from build123d import *

# Parameters (mm, degrees)
BOSS_EXTRUDE2_DEPTH = 50
CUT_EXTRUDE1_REACH  = 175.469
SKETCH2_W           = 5
SKETCH2_H           = 40
SKETCH3_W           = 40
SKETCH3_H           = 5
CUT_EXTRUDE4_DEPTH  = 25
CUT_EXTRUDE5_REACH  = 148.615
SKETCH5_W           = 40
SKETCH5_H           = 5
CUT_EXTRUDE6_REACH  = 175.469
SKETCH6_W           = 5
SKETCH6_H           = 40
FILLET1_R           = 10
FILLET2_R           = 3
FILLET3_R           = 8
CUT_EXTRUDE7_REACH  = 146.893
CUT_EXTRUDE8_DEPTH  = 145.893467036
SKETCH10_W          = 50
SKETCH10_H          = 14.886309014
CUT_EXTRUDE9_DEPTH  = 145.893467036
CUT_EXTRUDE10_REACH = 110.938
SKETCH11_R          = 6
CUT_EXTRUDE11_REACH = 144.895
SKETCH12_R          = 6


with BuildPart() as part:
    # Sketch1 → Boss-Extrude2 (new body)
    with BuildSketch(Plane.XY):
        Polygon((5, -20.716112532), (5, 136.021274565), (-55, 64.51605901), (-55, -20.716112532), (-45, -20.716112532), (-45, 60.876356667), (-5, 108.546500371), (-5, -20.716112532), align=None)
    extrude(amount=BOSS_EXTRUDE2_DEPTH)

    # Cut-Extrude1: up to this plane
    cut_extrude1_end = Plane(origin=(5, 136.021274565, 50), z_dir=(0.7660444431189773, -0.6427876096865403, 0))
    # Sketch2 → Cut-Extrude1 (cut, up to the surface)
    with BuildSketch(Plane.XZ.offset(20.716112532), mode=Mode.PRIVATE) as cut_extrude1_sk1:
        with Locations((-52.5, 25)):
            Rectangle(SKETCH2_W, SKETCH2_H)
    cut_extrude1_tool1 = split(extrude(cut_extrude1_sk1.sketch, amount=-CUT_EXTRUDE1_REACH, mode=Mode.PRIVATE), bisect_by=cut_extrude1_end, keep=Keep.BOTH, mode=Mode.PRIVATE)
    add(cut_extrude1_tool1.solids().sort_by_distance((-52.5, -20.716113, 25))[0], mode=Mode.SUBTRACT)

    # Sketch3 → Cut-Extrude4 (cut)
    with BuildSketch(Plane(origin=(14.043282439, 16.736132299, 0), x_dir=(0, 0, -1), z_dir=(0.6427876096865403, 0.7660444431189773, 0))):
        with Locations((-25, 81.102567729)):
            Rectangle(SKETCH3_W, SKETCH3_H)
    extrude(amount=-CUT_EXTRUDE4_DEPTH, mode=Mode.SUBTRACT)

    # Cut-Extrude5: up to this plane
    cut_extrude5_end = Plane(origin=(5, -20.716112532, 50), z_dir=(-1, 0, 0))
    # Sketch5 → Cut-Extrude5 (cut, up to the surface)
    with BuildSketch(Plane(origin=(14.043282439, 16.736132299, 0), x_dir=(0, 0, -1), z_dir=(0.6427876096865403, 0.7660444431189773, 0)), mode=Mode.PRIVATE) as cut_extrude5_sk1:
        with Locations((-25, 81.102567729)):
            Rectangle(SKETCH5_W, SKETCH5_H)
    cut_extrude5_tool1 = split(extrude(cut_extrude5_sk1.sketch, amount=CUT_EXTRUDE5_REACH, mode=Mode.PRIVATE), bisect_by=cut_extrude5_end, keep=Keep.BOTH, mode=Mode.PRIVATE)
    add(cut_extrude5_tool1.solids().sort_by_distance((-48.084889, 68.867858, 25))[0], mode=Mode.SUBTRACT)

    # Cut-Extrude6: up to this plane
    cut_extrude6_end = Plane(origin=(-62.239468027, 48.109777846, 45), z_dir=(0.7660444431189773, -0.6427876096865403, 0))
    # Sketch6 → Cut-Extrude6 (cut, up to the surface)
    with BuildSketch(Plane.XZ.offset(20.716112532), mode=Mode.PRIVATE) as cut_extrude6_sk1:
        with Locations((2.5, 25)):
            Rectangle(SKETCH6_W, SKETCH6_H)
    cut_extrude6_tool1 = split(extrude(cut_extrude6_sk1.sketch, amount=-CUT_EXTRUDE6_REACH, mode=Mode.PRIVATE), bisect_by=cut_extrude6_end, keep=Keep.BOTH, mode=Mode.PRIVATE)
    add(cut_extrude6_tool1.solids().sort_by_distance((2.5, -20.716113, 25))[0], mode=Mode.SUBTRACT)

    # Fillet1
    fillet1_edges = [part.edges().sort_by_distance(p)[0] for p in [
        (-45, 60.876356667, 25),
        (-55, 64.51605901, 47.5),
        (-55, 64.51605901, 2.5),
        (-50, 62.696207838, 25),
    ]]
    fillet(fillet1_edges, radius=FILLET1_R)

    # Fillet2
    fillet2_edges = [part.edges().sort_by_distance(p)[0] for p in [
        (-5, 108.546500371, 25),
        (0, 122.283887468, 25),
    ]]
    fillet(fillet2_edges, radius=FILLET2_R)

    # Fillet3
    fillet3_edges = [part.edges().sort_by_distance(p)[0] for p in [
        (5, 136.021274565, 47.5),
        (5, 136.021274565, 2.5),
    ]]
    fillet(fillet3_edges, radius=FILLET3_R)

    # Cut-Extrude7: up to this face of the body (flat: up to its plane)
    cut_extrude7_end = Plane(part.part.faces().sort_by_distance((5, 46.662671339, 2.5))[0])
    # Sketch8 → Cut-Extrude7 (cut, up to the picked face)
    with BuildSketch(Plane.ZY.offset(55), mode=Mode.PRIVATE) as cut_extrude7_sk1:
        Polygon((0, -20.716112532), (25, 19.170196482), (50, -20.716112532), align=None)
    cut_extrude7_tool1 = split(extrude(cut_extrude7_sk1.sketch, amount=-CUT_EXTRUDE7_REACH, mode=Mode.PRIVATE), bisect_by=cut_extrude7_end, keep=Keep.BOTH, mode=Mode.PRIVATE)
    add(cut_extrude7_tool1.solids().sort_by(Axis((-55, -7.420676, 25), (1, 0, 0)))[0], mode=Mode.SUBTRACT)

    # Sketch9 → Cut-Extrude8 (cut, through all)
    with BuildSketch(Plane(origin=(5, 0, 0), x_dir=(0, 0, -1), z_dir=(1, 0, 0))):
        Polygon((0, -5.829803518), (-25, 19.170196482), (-50, -5.829803518), align=None)
    extrude(amount=-CUT_EXTRUDE8_DEPTH, mode=Mode.SUBTRACT)


with BuildPart() as cut_extrude8_piece_1:
    # of the separate pieces the step leaves, piece 1, a body of its own (cut_extrude8_pieces)
    add(part.part.solids().sort_by_distance((-5, 100.304068112, 0))[0])

    # Sketch11 → Cut-Extrude10 (cut, up to next)
    with BuildSketch(Plane(origin=(-60.213060223, 50.524756626, 0), x_dir=(0, 0, 1), z_dir=(-0.7660444431189772, 0.6427876096865404, 0)), mode=Mode.PRIVATE) as cut_extrude10_sk1:
        with Locations(Location((25, 55.43246022, 0), (0, 0, 270))):
            Circle(SKETCH11_R)
    cut_extrude10_tool1 = extrude(cut_extrude10_sk1.sketch, amount=-CUT_EXTRUDE10_REACH, mode=Mode.PRIVATE) & cut_extrude8_piece_1.part
    add(cut_extrude10_tool1.solids().sort_by_distance((-24.581762, 92.988485, 25))[0], mode=Mode.SUBTRACT)

    # Sketch12 → Cut-Extrude11 (cut, up to next)
    with BuildSketch(Plane(origin=(0, 0, 0), x_dir=(0, 0, -1), z_dir=(1, 0, 0)), mode=Mode.PRIVATE) as cut_extrude11_sk1:
        with Locations((-25, 86.04145521)):
            Circle(SKETCH12_R)
    cut_extrude11_tool1 = extrude(cut_extrude11_sk1.sketch, amount=-CUT_EXTRUDE11_REACH, mode=Mode.PRIVATE) & cut_extrude8_piece_1.part
    add(cut_extrude11_tool1.solids().sort_by_distance((0, 86.041455, 25))[0], mode=Mode.SUBTRACT)


with BuildPart() as cut_extrude8_piece_2:
    # of the separate pieces the step leaves, piece 2, a body of its own (cut_extrude8_pieces)
    add(part.part.solids().sort_by_distance((-5, -20.716112532, 0))[0])


with BuildPart() as cut_extrude8_piece_3:
    # of the separate pieces the step leaves, piece 3, a body of its own (cut_extrude8_pieces)
    add(part.part.solids().sort_by_distance((-45, -20.716112532, 0))[0])


with BuildPart() as cut_extrude8_piece_4:
    # of the separate pieces the step leaves, piece 4, a body of its own (cut_extrude8_pieces)
    add(part.part.solids().sort_by_distance((-5, -20.716112532, 50))[0])


with BuildPart() as cut_extrude8_piece_5:
    # of the separate pieces the step leaves, piece 5, a body of its own (cut_extrude8_pieces)
    add(part.part.solids().sort_by_distance((-45, -20.716112532, 50))[0])


with BuildPart() as cut_extrude9_tool:
    # Sketch10 → Cut-Extrude9 (new, through all)
    with BuildSketch(Plane.ZY.offset(55)):
        with Locations((25, -13.272958025)):
            Rectangle(SKETCH10_W, SKETCH10_H)
    extrude(amount=-CUT_EXTRUDE9_DEPTH)


with BuildPart() as cut_extrude8_piece_2_1:
    add(cut_extrude8_piece_2.part)

    # Cut-Extrude9: cut by cut_extrude9_tool
    add(cut_extrude9_tool.part, mode=Mode.SUBTRACT)


with BuildPart() as cut_extrude8_piece_3_1:
    add(cut_extrude8_piece_3.part)

    # Cut-Extrude9: cut by cut_extrude9_tool
    add(cut_extrude9_tool.part, mode=Mode.SUBTRACT)


with BuildPart() as cut_extrude8_piece_4_1:
    add(cut_extrude8_piece_4.part)

    # Cut-Extrude9: cut by cut_extrude9_tool
    add(cut_extrude9_tool.part, mode=Mode.SUBTRACT)


with BuildPart() as cut_extrude8_piece_5_1:
    add(cut_extrude8_piece_5.part)

    # Cut-Extrude9: cut by cut_extrude9_tool
    add(cut_extrude9_tool.part, mode=Mode.SUBTRACT)


solid = cut_extrude8_piece_1.part
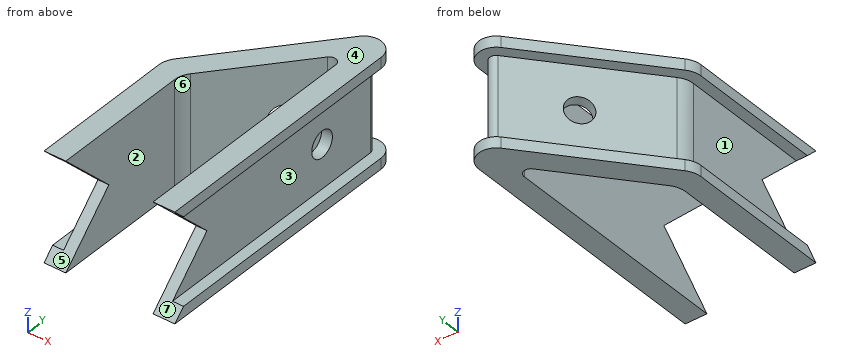
Read the model definition and answer for the solid it produces. Units are mm, in the model's axes. Face numbers are marked on the shaded views. A direction names the side the tool comes from. Round coordinates to 2 decimals unless told otherwise and drop trailing zeros. Order: outer loops, then holes, each group sorted by start corner. A loop starts at its lowest first (then second) coordinate and runs counter-clockwise, first axis right, second up.
1) Straight lines are drawn through the part: L1, parallel to X at y = 52.5, z = 26; L2, parallel to Z at x = -51.5, y = 57; L3, parallel to X at y = 37.5, z = 46. For each, find the intervals that lie inside material, in ascending order.
2) Flat-ended cylindrical pins translate along their axes: pin 1 (11 mm diameter, centred on y = 86.04, z = 25, fed in from -X); pin 2 (8 mm diameter, centred on x = -43.5, z = 14, fed in from +Y); pin 3 (1.5 mm diameter, centred on y = 50.5, z = 41.5, fed in from +X). Find the tip coordinate at first contact, or state that the pin passes through.
3) The part is cut by section C-C on y = 7. Write down the section's boundary in (x, z), plus the area to 3 significant figures.
4) The part is cut by section A-A on y = 32. Write down the section's boundary in (x, z), plus the area to 3 significant figures.
5) The part is cut by section B-B on z = 28.5. Write down the section's boundary in (x, y).
6) The mould has two halves that part along Z. Classify the marked faces 4, 5, 6 and 7: released by +Z, released by -Z, zero draft, split by the parting line, or undercut.
7) For the marked faces 1, 2 and 3, determine the directions among +Z, -Z, +X, -X, +Y, -Y from which every point of the face is accessible in a straight line to the end or side of a thin tool.
8) The part is cut by section D-D on x = -2. Write down the section's boundary in (y, z).
Resolved:
1. L1: x = -50 to -45, -5 to 0
1. L2: z = 0 to 5, 45 to 50
1. L3: x = -55 to -45, -5 to 5
2. pin 1: stops at x = -35.03
2. pin 2: stops at y = 75.21
2. pin 3: stops at x = 0
3. outline: (-55, 0) - (-45, 0) - (-45, 12.83) - (-50, 12.83) - (-50, 5) - (-55, 5) - close; (-55, 45) - (-50, 45) - (-50, 37.17) - (-45, 37.17) - (-45, 50) - (-55, 50) - close; (-5, 0) - (5, 0) - (5, 5) - (0, 5) - (0, 12.83) - (-5, 12.83) - close; (-5, 37.17) - (0, 37.17) - (0, 45) - (5, 45) - (5, 50) - (-5, 50) - close
3. area: 357 mm2
4. outline: (-55, 0) - (-45, 0) - (-45, 50) - (-55, 50) - (-55, 45) - (-50, 45) - (-50, 5) - (-55, 5) - close; (-5, 0) - (5, 0) - (5, 5) - (0, 5) - (0, 45) - (5, 45) - (5, 50) - (-5, 50) - close
4. area: 600 mm2
5. outline: (-50, 15.67) - (-45, 15.67) - (-45, 57.24) arc R10 cw to (-42.66, 63.66) - (-23.88, 86.04) - (-27.71, 89.26) - (-47.66, 65.48) arc R10 ccw to (-50, 59.06) - close; (-21.45, 96.72) - (-17.62, 93.51) - (-10.3, 102.23) arc R3 cw to (-5, 100.3) - (-5, 90.91) - (0, 90.91) - (0, 114.04) arc R3 ccw to (-5.3, 115.97) - close; (-5, 15.67) - (0, 15.67) - (0, 81.17) - (-5, 81.17) - close
6. face 4: released by +Z
6. face 5: undercut
6. face 6: zero draft
6. face 7: undercut
7. face 1: -X, +Y, -Y
7. face 2: +Z, -Z, -Y
7. face 3: +X, +Y, -Y
8. outline: (-5.83, 0) - (121.98, 0) - (121.98, 5) - (116.87, 5) - (116.87, 45) - (121.98, 45) - (121.98, 50) - (-5.83, 50) - (19.17, 25) - close; hole circle Ø12 at (86.04, 25)
